```python
from build123d import *

# Parameters (mm, degrees)
SKETCH1_R                = 90
BOSS_EXTRUDE1_DEPTH      = 101.5
CUT_EXTRUDE1_DEPTH       = 7.5
FILLET1_R                = 2
CIRPATTERN1_COUNT        = 4
FILLET1_OF_CIRPATTERN1_R = 2
SKETCH6_R                = 75
BOSS_EXTRUDE2_DEPTH      = 3
SKETCH7_R                = 57
BOSS_EXTRUDE3_DEPTH      = 3
SKETCH8_R                = 17.5
CUT_EXTRUDE2_DEPTH       = 10
SKETCH9_R                = 10
BOSS_EXTRUDE4_DEPTH      = 42
CUT_EXTRUDE3_START       = -20
CUT_EXTRUDE3_DEPTH       = 20
CUT_EXTRUDE4_DEPTH       = 167.698712469


with BuildPart() as part:
    # Sketch1 → Boss-Extrude1 (new body)
    with BuildSketch(Plane.XY):
        with Locations(Location((0, 0, 0), (0, 0, 180))):
            Circle(SKETCH1_R)
    extrude(amount=BOSS_EXTRUDE1_DEPTH)

    # Sketch2 → Cut-Extrude1 (cut)
    with BuildSketch(Plane(origin=(0, 0, 0), x_dir=(-1, 0, 0), z_dir=(0, 0, -1))):
        with BuildLine():
            Line((-5.15, 89.852531962), (-5.15, 85.15))
            ThreePointArc((-5.15, 85.15), (0, 80), (5.15, 85.15))
            Line((5.15, 85.15), (5.15, 89.852531962))
            ThreePointArc((5.15, 89.852531962), (0, 90), (-5.15, 89.852531962))
        make_face()
    cut_extrude1 = extrude(amount=-CUT_EXTRUDE1_DEPTH, mode=Mode.SUBTRACT)

    # Fillet1
    fillet1_edges = [part.edges().sort_by_distance(p)[0] for p in [
        (-5.15, 89.852531962, 3.75),
        (5.15, 89.852531962, 3.75),
    ]]
    fillet(fillet1_edges, radius=FILLET1_R)

    # Sketch5 → Tap Drill for M8 Tap1 (revolve, cut)
    with BuildSketch(Plane(origin=(-60.104076401, 60.104076401, 0), x_dir=(0, 1, 0), z_dir=(1, 0, 0))):
        Polygon((0, 0), (0, 15.5), (3.4, 13.457073895), (3.4, 0), align=None)
    tap_drill_for_m8_tap1 = revolve(axis=Axis((-60.104076401, 60.104076401, -6.35), (0, 0, 1)), mode=Mode.SUBTRACT)

    # CirPattern1: Cut-Extrude1, Tap Drill for M8 Tap1 ×4 about axis
    cirpattern1_axis = Axis((0, 0, 0), (0, 0, 1))
    add([cut_extrude1.rotate(cirpattern1_axis, i * 360 / CIRPATTERN1_COUNT) for i in range(1, CIRPATTERN1_COUNT)], mode=Mode.SUBTRACT)
    add([tap_drill_for_m8_tap1.rotate(cirpattern1_axis, i * 360 / CIRPATTERN1_COUNT) for i in range(1, CIRPATTERN1_COUNT)], mode=Mode.SUBTRACT)

    # Fillet1 of CirPattern1
    fillet1_of_cirpattern1_edges = [part.edges().sort_by_distance(p)[0] for p in [
        (-89.852531962, -5.15, 3.75),
        (-89.852531962, 5.15, 3.75),
        (5.15, -89.852531962, 3.75),
        (-5.15, -89.852531962, 3.75),
        (89.852531962, 5.15, 3.75),
        (89.852531962, -5.15, 3.75),
    ]]
    fillet(fillet1_of_cirpattern1_edges, radius=FILLET1_OF_CIRPATTERN1_R)

    # Sketch6 → Boss-Extrude2 (add)
    with BuildSketch(Plane(origin=(0, 0, 0), x_dir=(-1, 0, 0), z_dir=(0, 0, -1))):
        with Locations(Location((0, 0, 0), (0, 0, 180))):
            Circle(SKETCH6_R)
    extrude(amount=BOSS_EXTRUDE2_DEPTH)

    # Sketch7 → Boss-Extrude3 (add)
    with BuildSketch(Plane(origin=(0, 0, -3), x_dir=(-1, 0, 0), z_dir=(0, 0, -1))):
        Circle(SKETCH7_R)
    extrude(amount=BOSS_EXTRUDE3_DEPTH)

    # Sketch8 → Cut-Extrude2 (cut)
    with BuildSketch(Plane(origin=(0, 0, -6), x_dir=(-1, 0, 0), z_dir=(0, 0, -1))):
        Circle(SKETCH8_R)
    extrude(amount=-CUT_EXTRUDE2_DEPTH, mode=Mode.SUBTRACT)

    # Sketch9 → Boss-Extrude4 (add)
    with BuildSketch(Plane(origin=(0, 0, 4), x_dir=(-1, 0, 0), z_dir=(0, 0, -1))):
        with Locations(Location((0, 0, 0), (0, 0, 180))):
            Circle(SKETCH9_R)
    extrude(amount=BOSS_EXTRUDE4_DEPTH)

    # Sketch10 → Cut-Extrude3 (cut)
    with BuildSketch(Plane(origin=(0, 0, -38), x_dir=(-1, 0, 0), z_dir=(0, 0, -1)).offset(CUT_EXTRUDE3_START)):
        with BuildLine():
            Line((-2.5, 9.682458366), (-2.5, 6.882458366))
            Line((-2.5, 6.882458366), (2.5, 6.882458366))
            Line((2.5, 6.882458366), (2.5, 9.682458366))
            ThreePointArc((2.5, 9.682458366), (0, 10), (-2.5, 9.682458366))
        make_face()
    extrude(amount=CUT_EXTRUDE3_DEPTH, mode=Mode.SUBTRACT)

    # Sketch11 → Cut-Extrude4 (cut, through all)
    with BuildSketch(Plane(origin=(0, 6.882458366, 0), x_dir=(1, 0, 0), z_dir=(0, 1, 0))):
        with BuildLine():
            Line((2.5, 18), (-2.5, 18))
            ThreePointArc((-2.5, 18), (0, 15.5), (2.5, 18))
        make_face()
    extrude(amount=CUT_EXTRUDE4_DEPTH, mode=Mode.SUBTRACT)


solid = part.part
```
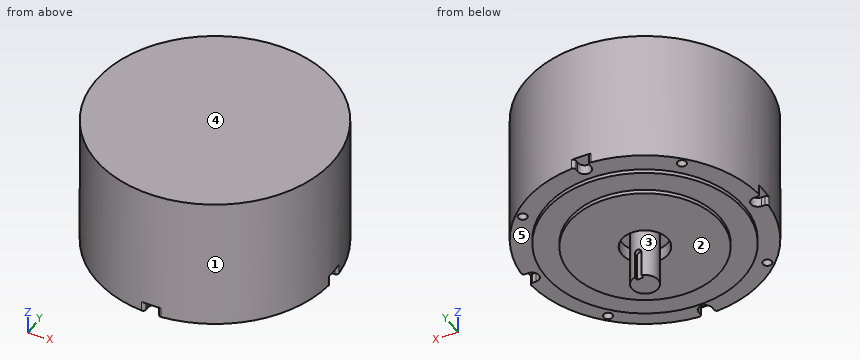
Input: part model. Units: mm. Frame: model coordinates. Face numbers are marked on the shaded views. A direction names the side the tool comes from. Give positions to 0.01 mm unless a question says otherwise; leave off trailing zeros. Order: outer loops, then holes, each group sorted by start corner. A loop starts at its lowest first (then second) coordinate and runs counter-clockwise, first axis right, second up. Notation, with made-up numbers: (88, 8.25) -> (144, 8.25) arc R12 ccw to (144, 19.25) -> close; hole circle Ø5 at (-5.5, 60.5). An arc over 180 degrees is marked (long way). Write each question's results on one line, items separated by ' | '. Start each with the question number.
Item 1: Line query: line 1 (Y direction, x = 0, z = 1.75); line 2 (Y direction, x = 3.5, z = -1.5); line 3 (Z direction, x = 5, y = -20). Output: solid intervals per line, ascending.
Item 2: Cut plane A-A on y = 0. Return the cut outline in (x, z), then the cut area to 3 significant figures.
Item 3: Cut plane B-B on x = 0. Return the cut outline in (y, z).
Item 4: Cut plane D-D on y = 72. Return the cut outline in (x, z), then the cut area to 3 significant figures.
Item 5: Contact query for flat-ended pins moving along their axis: P1, Ø8, axis at x = 35, z = 63, coming from the -Y side; P2, Ø5, axis at x = 11.5, z = 79.5, coming from the -Y side; P3, Ø6, axis at x = 46.5, z = 23, coming from the +Y side. Output: stop coordinate, or through.
Item 6: Mould query, pull axis Y, two halves, no side actions, for the marked faces 1, 2 and 3. Classes: pulls with the +Y half, pulls with the -Y half, needs draft (parallel to the pull), parting line crosses it, or undercut.
Item 7: Set-up query: the marked faces 4 and 5. Return all of +Z, -Z, +X, -X, +Y, -Y with unobstructed straight access to the full face (end or side cutting, diameter ignored); none if empty.
Item 8: Cut plane C-C on z = 42. Return the cut outline in (x, y), then the cut area to 3 significant figures.
Established:
1) line 1: -80 to -17.5, -10 to 10, 17.5 to 80 | line 2: -74.92 to -17.15, -9.37 to 9.37, 17.15 to 74.92 | line 3: -6 to 101.5
2) outline: (-90, 7.5) -> (-80, 7.5) -> (-80, 0) -> (-75, 0) -> (-75, -3) -> (-57, -3) -> (-57, -6) -> (-17.5, -6) -> (-17.5, 4) -> (-10, 4) -> (-10, -38) -> (10, -38) -> (10, 4) -> (17.5, 4) -> (17.5, -6) -> (57, -6) -> (57, -3) -> (75, -3) -> (75, 0) -> (80, 0) -> (80, 7.5) -> (90, 7.5) -> (90, 101.5) -> (-90, 101.5) -> close | area: 19,400 mm^2
3) outline: (-90, 7.5) -> (-80, 7.5) -> (-80, 0) -> (-75, 0) -> (-75, -3) -> (-57, -3) -> (-57, -6) -> (-17.5, -6) -> (-17.5, 4) -> (-10, 4) -> (-10, -38) -> (6.88, -38) -> (6.88, -15.5) -> (10, -15.5) -> (10, 4) -> (17.5, 4) -> (17.5, -6) -> (57, -6) -> (57, -3) -> (75, -3) -> (75, 0) -> (80, 0) -> (80, 7.5) -> (90, 7.5) -> (90, 101.5) -> (-90, 101.5) -> close
4) outline: (-54, 0) -> (-21, 0) -> (-21, -3) -> (21, -3) -> (21, 0) -> (54, 0) -> (54, 101.5) -> (-54, 101.5) -> close | area: 11,100 mm^2
5) P1: y = -84.49 | P2: y = -89.55 | P3: y = 78.79
6) face 1: parting line crosses it | face 2: needs draft | face 3: undercut
7) face 4: +Z, +X, -X, +Y, -Y | face 5: -Z
8) outline: circle Ø180 at (0, 0) | area: 25,400 mm^2
